The model under review builds one solid part; all positions refer to its coordinate system, in mm. Coordinates: 2 decimals unless noted, no trailing zeros. Order: outer loops, then holes, each group sorted by start corner. A loop starts at its lowest first (then second) coordinate and runs counter-clockwise, first axis right, second up. Notation, with made-up numbers: M 8.5,73 L 22.5,73 A20 cw 22.5,84 Z; hole C 14.25,89.25 d10. An arc over 180 degrees is marked long. Answer as CSV lines item,"result". Start each with the question number.
Q1. Consider section A-A on z = -47. Write out the cut boundary in (x, y).
Q2. Consider section B-B on x = 5.5. Write out the cut boundary in (y, z), and give its area (3 significant figures).
Q3. Wall thickness on L1, parallel to X at y = 0.85, z = 0.5; L2, parallel to Z at x = 9, y = 0.4; L3, parallel to Z at x = -20, y = 0.1: over which ranges is each line inside the solid? List them lowest first. Write a range as [from, to].
Q4. Consider section C-C on x = 24.5. Write out the cut boundary in (y, z), and give its area (3 significant figures).
Q5. For P1, Ø0.5, axis at y = 0.5, z = -74, coming from the +X side; P2, Ø0.5, axis at x = -5.5, y = 0.5, coming from the -Z side; P3, Ø0.5, axis at y = 0.5, z = -1, coming from the -X side; P4, Ø12, axis at x = -4.5, z = -71.5, coming from the +Y side, all flat-tipped, find the tip position at first contact; note any pin that passes through.
from build123d import *

# Parameters (mm, degrees)
EXTRUDE_3_DEPTH          = 1
EXTRUDE_3_2_DEPTH        = 1
CUT_EXTRUDE_3_DEPTH      = 2
CUT_EXTRUDE_3_DEPTH_BACK = 2
SKETCH_3_W               = 1
SKETCH_3_H               = 57.878930007
SKETCH_4_W               = 1
SKETCH_4_H               = 165.358983849
EXTRUDE_4_DEPTH          = 1


with BuildPart() as part:
    # Sketch 2 → Extrude 3 (new body)
    with BuildSketch(Plane(origin=(0, 0, 0), x_dir=(1, 0, 0), z_dir=(0, 1, 0))):
        with BuildLine():
            Line((28.5, 19.918584287), (20.577350269, 33.641016151))
            ThreePointArc((20.577350269, 33.641016151), (19.845299462, 34.373066959), (18.845299462, 34.641016151))
            Line((18.845299462, 34.641016151), (-18.845299462, 34.641016151))
            ThreePointArc((-18.845299462, 34.641016151), (-19.845299462, 34.373066959), (-20.577350269, 33.641016151))
            Line((-20.577350269, 33.641016151), (-28.5, 19.918584287))
            ThreePointArc((-28.5, 19.918584287), (-28.699800845, 18.400946197), (-27.767949192, 17.186533479))
            Line((-27.767949192, 17.186533479), (0, 1.154700538))
            Line((0, 1.154700538), (27.767949192, 17.186533479))
            ThreePointArc((27.767949192, 17.186533479), (28.699800845, 18.400946197), (28.5, 19.918584287))
        make_face()
        with BuildLine():
            Line((15.958548116, 29.641016151), (-15.958548116, 29.641016151))
            ThreePointArc((-15.958548116, 29.641016151), (-16.958548116, 29.373066959), (-17.690598923, 28.641016151))
            Line((-17.690598923, 28.641016151), (-21.669872981, 21.748711306))
            ThreePointArc((-21.669872981, 21.748711306), (-21.869673826, 20.231073216), (-20.937822174, 19.016660498))
            Line((-20.937822174, 19.016660498), (0, 6.92820323))
            Line((0, 6.92820323), (21.026102441, 19.067629134))
            ThreePointArc((21.026102441, 19.067629134), (21.910458886, 20.220144892), (21.720841617, 21.660431039))
            Line((21.720841617, 21.660431039), (17.690598923, 28.641016151))
            ThreePointArc((17.690598923, 28.641016151), (16.958548116, 29.373066959), (15.958548116, 29.641016151))
        make_face(mode=Mode.SUBTRACT)
    extrude(amount=EXTRUDE_3_DEPTH)


with BuildPart() as body_2:
    # Sketch 2 → Extrude 3 2 (new body)
    with BuildSketch(Plane(origin=(0, 0, 0), x_dir=(1, 0, 0), z_dir=(0, 1, 0))):
        with BuildLine():
            Line((-28.550968636, -19.83030402), (-20.547923514, -33.691984787))
            ThreePointArc((-20.547923514, -33.691984787), (-19.853184337, -34.386723964), (-18.904152973, -34.641016151))
            Line((-18.904152973, -34.641016151), (18.904152973, -34.641016151))
            ThreePointArc((18.904152973, -34.641016151), (19.853184337, -34.386723964), (20.547923514, -33.691984787))
            Line((20.547923514, -33.691984787), (28.550968636, -19.83030402))
            ThreePointArc((28.550968636, -19.83030402), (28.740585904, -18.390017873), (27.856229459, -17.237502115))
            Line((27.856229459, -17.237502115), (0, -1.154700538))
            Line((0, -1.154700538), (-27.856229459, -17.237502115))
            ThreePointArc((-27.856229459, -17.237502115), (-28.740585904, -18.390017873), (-28.550968636, -19.83030402))
        make_face()
        with BuildLine():
            Line((-21.026102441, -19.067629134), (0, -6.92820323))
            Line((0, -6.92820323), (21.026102441, -19.067629134))
            ThreePointArc((21.026102441, -19.067629134), (21.910458886, -20.220144892), (21.720841617, -21.660431039))
            Line((21.720841617, -21.660431039), (17.661172168, -28.691984787))
            ThreePointArc((17.661172168, -28.691984787), (16.966432991, -29.386723964), (16.017401627, -29.641016151))
            Line((16.017401627, -29.641016151), (-16.017401627, -29.641016151))
            ThreePointArc((-16.017401627, -29.641016151), (-16.966432991, -29.386723964), (-17.661172168, -28.691984787))
            Line((-17.661172168, -28.691984787), (-21.720841617, -21.660431039))
            ThreePointArc((-21.720841617, -21.660431039), (-21.910458886, -20.220144892), (-21.026102441, -19.067629134))
        make_face(mode=Mode.SUBTRACT)
    extrude(amount=EXTRUDE_3_2_DEPTH)


with BuildPart() as cut_extrude_3_tool:
    # Sketch 3 → Cut-Extrude 3 (new, two sides: drawn at the far end of the back side and taken through both)
    with BuildSketch(Plane(origin=(0, 0, 0), x_dir=(1, 0, 0), z_dir=(0, 1, 0)).offset(-CUT_EXTRUDE_3_DEPTH_BACK)):
        with Locations((0, 6.92820323)):
            Rectangle(SKETCH_3_W, SKETCH_3_H)
    extrude(amount=CUT_EXTRUDE_3_DEPTH + CUT_EXTRUDE_3_DEPTH_BACK)


with BuildPart() as part_1:
    add(part.part)

    # Cut-Extrude 3: cut by cut_extrude_3_tool
    add(cut_extrude_3_tool.part, mode=Mode.SUBTRACT)



with BuildPart() as body_2_1:
    add(body_2.part)

    # Cut-Extrude 3: cut by cut_extrude_3_tool
    add(cut_extrude_3_tool.part, mode=Mode.SUBTRACT)


with BuildPart() as part_2:
    add(part_1.part)

    add(body_2_1.part)  # Extrude 4 merges body 2
    # Sketch 4 → Extrude 4 (add)
    with BuildSketch(Plane(origin=(0, 0, 0), x_dir=(1, 0, 0), z_dir=(0, 1, 0))):
        Polygon((-1.5, 2.020725942), (-1.5, -2.020725942), (-0.5, -1.443375673), (-0.5, 1.443375673), align=None)
        Polygon((0.5, 1.443375673), (0.5, -1.443375673), (1.5, -2.020725942), (1.5, 2.020725942), align=None)
        with Locations((-1, 117.320508076)):
            Rectangle(SKETCH_4_W, SKETCH_4_H)
        with Locations((1, 117.320508076)):
            Rectangle(SKETCH_4_W, SKETCH_4_H)
    extrude(amount=EXTRUDE_4_DEPTH)


solid = part_2.part
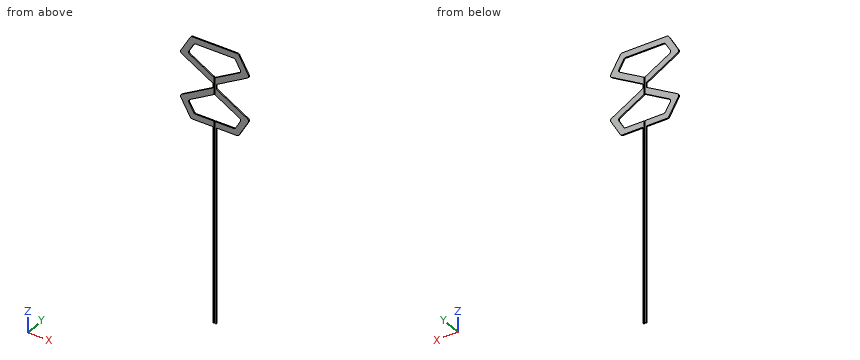
Evaluation:
1,outline,"M -1.5,0 L -0.5,0 L -0.5,1 L -1.5,1 Z; M 0.5,0 L 1.5,0 L 1.5,1 L 0.5,1 Z"
2,outline,"M 0,-34.64 L 1,-34.64 L 1,-29.64 L 0,-29.64 Z; M 0,-10.1 L 1,-10.1 L 1,-4.33 L 0,-4.33 Z; M 0,4.33 L 1,4.33 L 1,10.1 L 0,10.1 Z; M 0,29.64 L 1,29.64 L 1,34.64 L 0,34.64 Z"
2,area,"21.5 mm²"
3,L1,"x = [-1.5, -0.5], [0.5, 1.5]"
3,L2,"z = [-34.64, -29.64], [-12.12, -6.35], [6.35, 12.12], [29.64, 34.64]"
3,L3,"z = [-34.27, -24.64], [-18.48, -12.7], [12.7, 18.48], [24.64, 34.29]"
4,outline,"M 0,-26.85 L 1,-26.85 L 1,-15.3 L 0,-15.3 Z; M 0,15.3 L 1,15.3 L 1,26.85 L 0,26.85 Z"
4,area,"23.1 mm²"
5,P1,"stops at x = 1.5"
5,P2,"stops at z = -34.64"
5,P3,"stops at x = -1.5"
5,P4,"stops at y = 1"
